The figure shows three views and two pictorial views of one solid part (mm, origin at its lowest corner). Answer the questions. A direction names the side the tool comes from. Give positions to 0.01 mm unless a question says otherwise; leave off trailing zeros. Order: outer loops, then holes, each group sorted by start corner. A loop starts at its lowest first (then second) coordinate and runs counter-clockwise, first axis right, second up. Notation, with made-up numbers: (13.5, 58.5) - (59.5, 58.5) arc R32 ccw to (59.5, 95.5) - close; hole circle Ø5 at (64.5, 4). An arc over 180 degrees is marked (long way). Return JSON: item names as keys, results as strings. Group by question number.
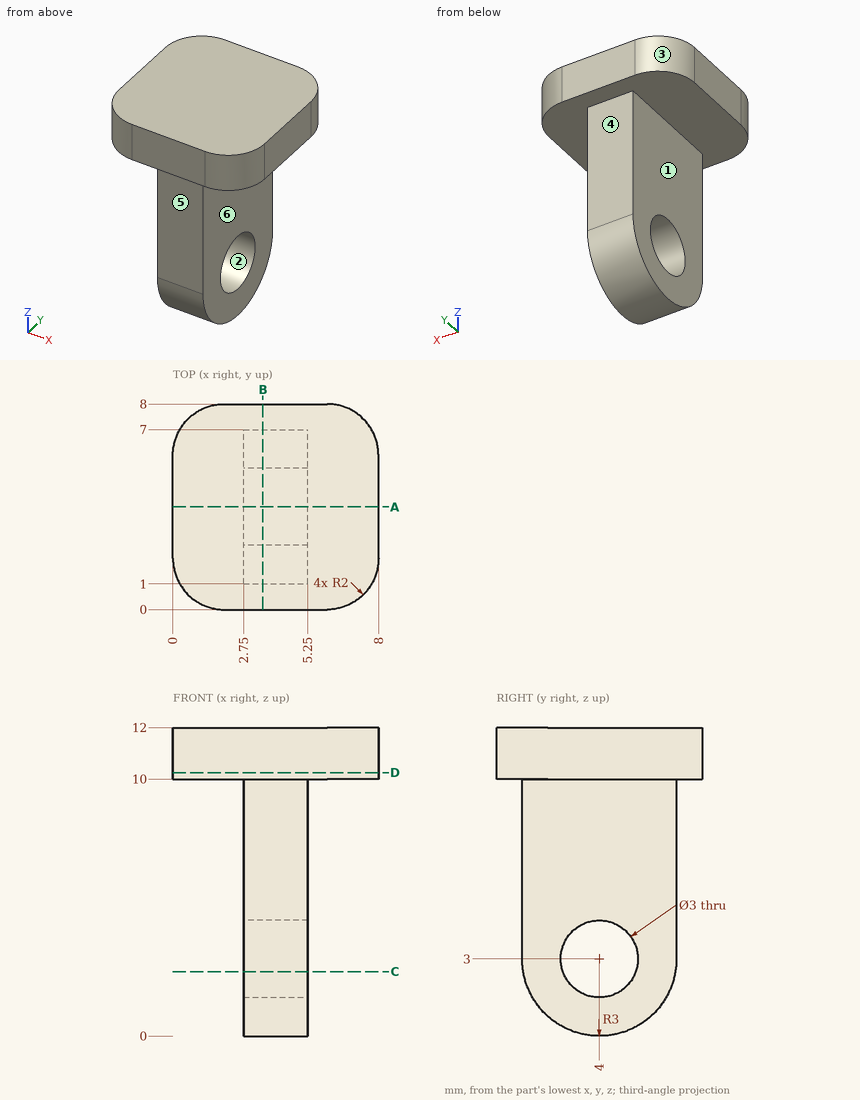
1. Each of these flat-tipped pins is pushed along its axis until it touches: pin 1 (3 mm diameter, centred on x = 4, z = 7, fed in from +Y); pin 2 (2 mm diameter, centred on x = 3.5, z = 6, fed in from -Y); pin 3 (1.5 mm diameter, centred on y = 5.5, z = 5, fed in from -X). Where does it stop, or does it pass through?
2. Determine the mould class of the marked faces 1, 2 and 3 for opening direction Y: released by +Y, released by -Y, zero draft, split by the parting line, or undercut.
3. The part is cut by section C-C (z = 2.5). Give the vertices of the cut face in (x, y).
4. A tool of negligible diameter and unlimited length cuts with its end or side. For the marked faces 4, 5 and 6, from which of +Z, -Z, +X, -X, +Y, -Y can it reach the whole face along a straight path? Write none if from no direction.
5. The part is cut by section A-A (y = 4). Give the vertices of the cut face in (x, z).
6. The part is cut by section B-B (x = 3.5). Give the vertices of the cut face in (y, z), and give its area (3 significant figures).
7. Consider probe 1 along Z at (x, y) = (3.5, 4); probe 2 along Y at (x, z) = (4.5, 3); probe 3 along Z at (x, y) = (5.75, 5.5). Determine where each line is inside the solid, lowest interval first. Write a range as from..to.
8. The part is cut by section D-D (z = 10.25). Give the vertices of the cut face in (x, y).
Answers:
{
 "1": {"pin 1": "stops at y = 7", "pin 2": "stops at y = 1", "pin 3": "stops at x = 2.75"},
 "2": {"face 1": "zero draft", "face 2": "undercut", "face 3": "released by +Y"},
 "3": {"outline": "(2.75, 1.04) - (5.25, 1.04) - (5.25, 2.59) - (2.75, 2.59) - close; (2.75, 5.41) - (5.25, 5.41) - (5.25, 6.96) - (2.75, 6.96) - close"},
 "4": {"face 4": "-Z, +X, -X, +Y", "face 5": "-Z, +X, -X, -Y", "face 6": "-Z, +X, +Y, -Y"},
 "5": {"outline": "(0, 10) - (2.75, 10) - (2.75, 4.5) - (5.25, 4.5) - (5.25, 10) - (8, 10) - (8, 12) - (0, 12) - close; (2.75, 0) - (5.25, 0) - (5.25, 1.5) - (2.75, 1.5) - close"},
 "6": {"outline": "(0, 10) - (1, 10) - (1, 3) arc R3 ccw to (7, 3) - (7, 10) - (8, 10) - (8, 12) - (0, 12) - close; hole circle Ø3 at (4, 3)", "area": "65.1 mm^2"},
 "7": {"probe 1": "z = 0..1.5, 4.5..12", "probe 2": "y = 1..2.5, 5.5..7", "probe 3": "z = 10..12"},
 "8": {"outline": "(0, 2) arc R2 ccw to (2, 0) - (6, 0) arc R2 ccw to (8, 2) - (8, 6) arc R2 ccw to (6, 8) - (2, 8) arc R2 ccw to (0, 6) - close"}
}
